```python
from build123d import *

# Parameters (mm, degrees)
SKETCH_1_W          = 42
SKETCH_1_H          = 48
SKETCH_1_R          = 1.25
EXTRUDE_1_DEPTH     = 15
SKETCH_2_R          = 3
SKETCH_2_R_2        = 1.25
CUT_EXTRUDE_1_DEPTH = 20


with BuildPart() as part:
    # 草圖1 → 填料-伸長1 (new body)
    with BuildSketch(Plane.XY):
        with Locations((-20.813738939, -9.020397992)):
            Rectangle(SKETCH_1_W, SKETCH_1_H)
        with Locations((-36.813738939, 5.979602008)):
            Circle(SKETCH_1_R, mode=Mode.SUBTRACT)
        with Locations((-36.813738939, -20.020397992)):
            Circle(SKETCH_1_R, mode=Mode.SUBTRACT)
        with Locations((-4.813738939, -20.020397992)):
            Circle(SKETCH_1_R, mode=Mode.SUBTRACT)
        with Locations((-4.813738939, 5.979602008)):
            Circle(SKETCH_1_R, mode=Mode.SUBTRACT)
    extrude(amount=EXTRUDE_1_DEPTH)

    # 草圖2 → 除料-伸長1 (cut)
    with BuildSketch(Plane.XY.offset(15)):
        with Locations((-20.813738939, -21.020397992)):
            Circle(SKETCH_2_R)
        with Locations((-20.813738939, -14.020397992)):
            Circle(SKETCH_2_R_2)
        with Locations((-25.763486407, -16.070650524)):
            Circle(SKETCH_2_R_2)
        with Locations((-27.813738939, -21.020397992)):
            Circle(SKETCH_2_R_2)
        with Locations((-25.763486407, -25.970145461)):
            Circle(SKETCH_2_R_2)
        with Locations((-20.813738939, -28.020397992)):
            Circle(SKETCH_2_R_2)
        with Locations((-15.86399147, -25.970145461)):
            Circle(SKETCH_2_R_2)
        with Locations((-13.813738939, -21.020397992)):
            Circle(SKETCH_2_R_2)
        with Locations((-15.86399147, -16.070650524)):
            Circle(SKETCH_2_R_2)
    extrude(amount=-CUT_EXTRUDE_1_DEPTH, mode=Mode.SUBTRACT)


solid = part.part
```
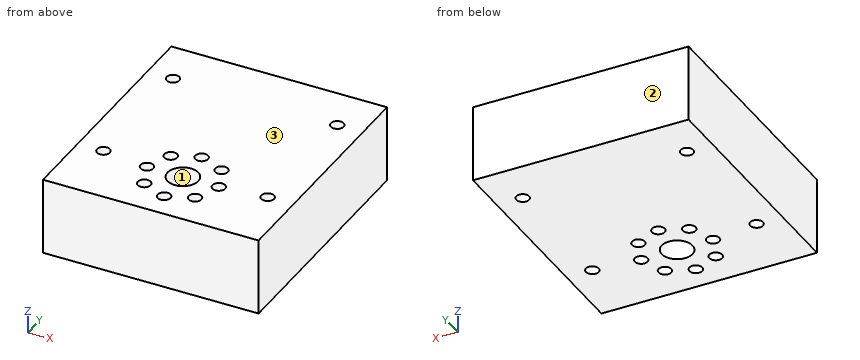
Part model, mm, in its own coordinate system. Face numbers are marked on the shaded views. Coordinates: 2 decimals unless noted, no trailing zeros. Loops run counter-clockwise (first coordinate to the right, second up) from the corner with the lowest first, then second, coordinate; pieces in that order, holes last. Notation, with made-up numbers: (0, 37) - (12, 37) arc R11 ccw to (12, 51) - close; hole circle Ø5 at (-31, -16.75). An arc over 180 degrees is marked (long way). Write item = value, one per line. Start each with the question number.
Item 1: Cut at D-D, the plane x = -14. Give the cut face in (y, z).
Item 2: Mould opens along Y. For the marked faces 1, 2 and 3 say: released by +Y, released by -Y, zero draft, split by the parting line, or undercut.
Item 3: Cut at B-B, the plane x = -19. Give the cut face in (y, z), and give its area (3 significant figures).
Item 4: Cut at A-A, the plane x = -4.5. Give the cut face in (y, z), and give its area (3 significant figures).
Item 5: Wall check: L1, parallel to X at y = 6, z = 6; L2, parallel to X at y = -22, z = 12.25; L3, parallel to Y at x = -5.5, z = 11.75. Give the ranges that are in metal, low to high. Write a range as from..to.
Item 6: Cut at C-C, the plane z = 11.75. State how many separate pieces and enclosed holes the cut face has, and give its area (3 significant figures).
Item 7: Flat gauge pin, fed straight in: pin 1 Ø4 at (x, y) = (-36.81, 5.98) entering from +Z. Where does the tip first touch, or does it go through?
The answers:
q1.outline = (-33.02, 0) - (-22.26, 0) - (-22.26, 15) - (-33.02, 15) - close; (-19.78, 0) - (14.98, 0) - (14.98, 15) - (-19.78, 15) - close
q2.face_1 = undercut
q2.face_2 = released by +Y
q2.face_3 = zero draft
q3.outline = (-33.02, 0) - (-23.41, 0) - (-23.41, 15) - (-33.02, 15) - close; (-18.63, 0) - (14.98, 0) - (14.98, 15) - (-18.63, 15) - close
q3.area = 648 mm2
q4.outline = (-33.02, 0) - (-21.23, 0) - (-21.23, 15) - (-33.02, 15) - close; (-18.81, 0) - (4.77, 0) - (4.77, 15) - (-18.81, 15) - close; (7.19, 0) - (14.98, 0) - (14.98, 15) - (7.19, 15) - close
q4.area = 647 mm2
q5.L1 = -41.81..-38.06, -35.56..-6.06, -3.56..0.19
q5.L2 = -41.81..-28.59, -27.04..-23.65, -17.98..-14.59, -13.04..0.19
q5.L3 = -33.02..-21.07, -18.98..4.93, 7.02..14.98
q6.separate_pieces = 1
q6.enclosed_holes = 13
q6.area = 1,930 mm2
q7.pin_1 = 15
